Can you work these out from the model? Positions are in its coordinate system, mm. A direction names the side the tool comes from. Give positions to 0.01 mm unless a question says otherwise; leave off trailing zeros. Write each loop counter-clockwise with the first axis right and the second up, starting at its lowest first coordinate (ties: lowest second). Pieces come first, ordered by that corner, then holes.
from build123d import *

# Parameters (mm, degrees)
SKETCH1_W           = 44.958
SKETCH1_H           = 304.8
BOSS_EXTRUDE1_DEPTH = 5.588
SKETCH2_W           = 5.588
SKETCH2_H           = 101.6
BOSS_EXTRUDE2_DEPTH = 5.588
SKETCH3_W           = 222.25
SKETCH3_H           = 5.588
BOSS_EXTRUDE3_DEPTH = 39.37
SKETCH7_W           = 327.022738736
SKETCH7_H           = 279.435650021
CUT_EXTRUDE1_DEPTH  = 45.958
SKETCH4_W           = 6.35
SKETCH4_H           = 5.588
SKETCH4_H_2         = 12.7
CUT_EXTRUDE2_DEPTH  = 5.588
SKETCH6_W           = 5.588
SKETCH6_H           = 16.933333333
SKETCH6_H_2         = 16.933333334
CUT_EXTRUDE3_DEPTH  = 6.588
SKETCH8_W           = 9.525
SKETCH8_H           = 25.4
BOSS_EXTRUDE4_DEPTH = 5.588


with BuildPart() as part:
    # Sketch1 → Boss-Extrude1 (new body)
    with BuildSketch(Plane.XY):
        with Locations((-6.477, 3.048)):
            Rectangle(SKETCH1_W, SKETCH1_H)
        with BuildLine():
            Line((-3.302, 133.858), (-3.302, -143.002))
            Line((-3.302, -143.002), (3.302, -143.002))
            Line((3.302, -143.002), (3.302, 143.002))
            Line((3.302, 143.002), (-16.256, 143.002))
            Line((-16.256, 143.002), (-16.256, 136.398))
            Line((-16.256, 136.398), (-5.842, 136.398))
            ThreePointArc((-5.842, 136.398), (-4.045948776, 135.654051224), (-3.302, 133.858))
        make_face(mode=Mode.SUBTRACT)
    extrude(amount=BOSS_EXTRUDE1_DEPTH)

    # Sketch2 → Boss-Extrude2 (add)
    with BuildSketch(Plane(origin=(16.002, 0, 0), x_dir=(0, 0, -1), z_dir=(1, 0, 0))):
        Polygon((222.25, -60.452), (222.25, -47.752), (0, -47.752), (0, -149.352), (222.25, -149.352), (222.25, -136.652), (228.6, -136.652), (228.6, -119.718666667), (222.25, -119.718666667), (222.25, -107.018666667), (228.6, -107.018666667), (228.6, -90.085333333), (222.25, -90.085333333), (222.25, -77.385333333), (228.6, -77.385333333), (228.6, -60.452), align=None)
        with BuildLine():
            ThreePointArc((11.4, -116.592), (9.9, -118.092), (8.4, -116.592))
            Line((8.4, -116.592), (8.4, -111.512))
            ThreePointArc((8.4, -111.512), (9.9, -110.012), (11.4, -111.512))
            Line((11.4, -111.512), (11.4, -116.592))
        make_face(mode=Mode.SUBTRACT)
        with BuildLine():
            Line((42.4, -111.512), (42.4, -116.592))
            ThreePointArc((42.4, -116.592), (40.9, -118.092), (39.4, -116.592))
            Line((39.4, -116.592), (39.4, -111.512))
            ThreePointArc((39.4, -111.512), (40.9, -110.012), (42.4, -111.512))
        make_face(mode=Mode.SUBTRACT)
        with BuildLine():
            ThreePointArc((36.4, -101.092), (25.4, -112.092), (14.4, -101.092))
            Line((14.4, -101.092), (14.4, -96.012))
            ThreePointArc((14.4, -96.012), (25.4, -85.012), (36.4, -96.012))
            Line((36.4, -96.012), (36.4, -101.092))
        make_face(mode=Mode.SUBTRACT)
        with BuildLine():
            ThreePointArc((11.4, -85.592), (9.9, -87.092), (8.4, -85.592))
            Line((8.4, -85.592), (8.4, -80.512))
            ThreePointArc((8.4, -80.512), (9.9, -79.012), (11.4, -80.512))
            Line((11.4, -80.512), (11.4, -85.592))
        make_face(mode=Mode.SUBTRACT)
        with BuildLine():
            ThreePointArc((42.4, -85.592), (40.9, -87.092), (39.4, -85.592))
            Line((39.4, -85.592), (39.4, -80.512))
            ThreePointArc((39.4, -80.512), (40.9, -79.012), (42.4, -80.512))
            Line((42.4, -80.512), (42.4, -85.592))
        make_face(mode=Mode.SUBTRACT)
        with Locations((-2.794, -98.552)):
            Rectangle(SKETCH2_W, SKETCH2_H)
    extrude(amount=-BOSS_EXTRUDE2_DEPTH)

    # Sketch3 → Boss-Extrude3 (add)
    with BuildSketch(Plane.ZY.offset(-10.414)):
        with Locations((-111.125, -146.558)):
            Rectangle(SKETCH3_W, SKETCH3_H)
    extrude(amount=BOSS_EXTRUDE3_DEPTH)

    # Sketch7 → Cut-Extrude1 (cut, through all)
    with BuildSketch(Plane(origin=(16.002, 0, 0), x_dir=(0, 0, -1), z_dir=(1, 0, 0))):
        with Locations((163.511369368, -148.348068682)):
            Rectangle(SKETCH7_W, SKETCH7_H)
    extrude(amount=-CUT_EXTRUDE1_DEPTH, mode=Mode.SUBTRACT)

    # Sketch4 → Cut-Extrude2 (cut)
    with BuildSketch(Plane.XZ.offset(149.352)):
        with Locations((-12.954, 2.794)):
            Rectangle(SKETCH4_W, SKETCH4_H)
        with Locations((12.827, 2.794)):
            Rectangle(SKETCH4_W, SKETCH4_H)
        with Locations((-25.781, 2.794)):
            Rectangle(SKETCH4_W, SKETCH4_H)
        with Locations((12.827, -135.22325)):
            Rectangle(SKETCH4_W, SKETCH4_H_2)
        with Locations((12.827, -54.5465)):
            Rectangle(SKETCH4_W, SKETCH4_H_2)
        with Locations((12.827, -162.1155)):
            Rectangle(SKETCH4_W, SKETCH4_H_2)
    extrude(amount=-CUT_EXTRUDE2_DEPTH, mode=Mode.SUBTRACT)

    # Sketch6 → Cut-Extrude3 (cut, through all)
    with BuildSketch(Plane.XY.offset(5.588)):
        with Locations((13.208, -68.918666667)):
            Rectangle(SKETCH6_W, SKETCH6_H)
        with Locations((13.208, -98.552)):
            Rectangle(SKETCH6_W, SKETCH6_H_2)
        with Locations((13.208, -128.185333334)):
            Rectangle(SKETCH6_W, SKETCH6_H)
    extrude(amount=-CUT_EXTRUDE3_DEPTH, mode=Mode.SUBTRACT)

    # Sketch8 → Boss-Extrude4 (add)
    with BuildSketch(Plane.XY.offset(5.588)):
        with Locations((-33.7185, 133.477)):
            Rectangle(SKETCH8_W, SKETCH8_H)
        with Locations((20.7645, 133.477)):
            Rectangle(SKETCH8_W, SKETCH8_H)
    extrude(amount=-BOSS_EXTRUDE4_DEPTH)


solid = part.part
(1) Imagine slicing it at A-A, the plane y = 125.5. Write out the boundary of the cut face in (x, z), plus the area to 3 significant figures.
Returned:
outline: (-38.48, 0) - (-3.3, 0) - (-3.3, 5.59) - (-38.48, 5.59) - close; (3.3, 0) - (25.53, 0) - (25.53, 5.59) - (3.3, 5.59) - close
area: 321 mm2
(2) Imagine slicing it at B-B, the plane x = 0.5. Write out the boundary of the cut face in (y, z), plus the area to 3 significant figures.
Returned:
outline: (-149.35, 0) - (-143, 0) - (-143, 5.59) - (-149.35, 5.59) - close; (143, 0) - (155.45, 0) - (155.45, 5.59) - (143, 5.59) - close
area: 105 mm2
(3) Will these pins go through, and if not, where does the flat tip stop? P1, Ø3, axis at x = -34.5, z = 2, coming from the -Y side; P2, Ø3, axis at y = -112.5, z = 2.5, coming from the +X side; P3, Ø3, axis at y = 150, z = 2, coming from the -X side.
Returned:
P1: stops at y = 120.78
P2: stops at x = 16
P3: stops at x = -28.96
(4) If I drill on L1, parallel to X at y = 15, z = 4.6; L2, parallel to Y at x = -14, z = 4.8; L3, parallel to Y at x = 13.5, z = 3.9, over which ranges is the centre line in solid material (lowest first)?
Returned:
L1: x = -28.96 to -3.3, 3.3 to 16
L2: y = -143.76 to 136.4, 143 to 155.45
L3: y = -143.76 to -136.65, -119.72 to -107.02, -90.09 to -77.39, -60.45 to 155.45
(5) For faces 1 (the face through (10.414, -128, 3)), 2 (the face through (-34, 120.777, 3)), 3 (the face through (16.002, -140, 3)), which set-ups out of +Z, -Z, +X, -X, +Y, -Y let a thin tool reach every point of the face, with its end or its side?
Returned:
face 1: +Z, -Z, +X
face 2: +Z, -Z, -X, -Y
face 3: +Z, -Z, +X, -Y
